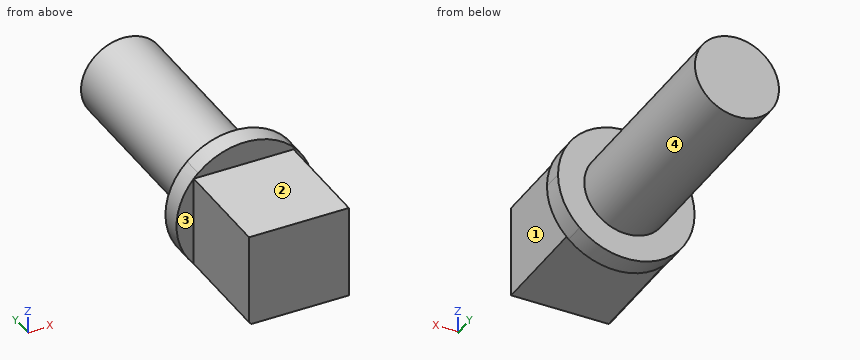
```python
from build123d import *

# Parameters (mm, degrees)
F0_R     = 4
F1_DEPTH = 22
F0_W     = 8.8741196746
F0_H     = 9.5
F2_DEPTH = 2
F3_DEPTH = 10
F5_DEPTH = 10


with BuildPart() as f1:
    # F0 (on Front) → F1 (new body)
    with BuildSketch(Plane.XZ):
        Circle(F0_R)
    extrude(amount=-F1_DEPTH)

    # F0 (on Front) → F2 (join)
    with BuildSketch(Plane.XZ):
        with BuildLine():
            ThreePointArc((4.4370598373, -4.75), (5.9620000395, -2.5893156487), (6.5, 0))
            ThreePointArc((6.5, 0), (5.9620000395, 2.5893156487), (4.4370598373, 4.75))
            Line((4.4370598373, 4.75), (4.4370598373, -4.75))
        make_face()
        with BuildLine():
            Line((-4.4370598373, 4.75), (4.4370598373, 4.75))
            ThreePointArc((4.4370598373, 4.75), (0, 6.5), (-4.4370598373, 4.75))
        make_face()
        Rectangle(F0_W, F0_H)
        Circle(F0_R, mode=Mode.SUBTRACT)
        with BuildLine():
            ThreePointArc((-4.4370598373, -4.75), (0, -6.5), (4.4370598373, -4.75))
            Line((4.4370598373, -4.75), (-4.4370598373, -4.75))
        make_face()
        with BuildLine():
            Line((-4.4370598373, -4.75), (-4.4370598373, 4.75))
            ThreePointArc((-4.4370598373, 4.75), (-6.5, 0), (-4.4370598373, -4.75))
        make_face()
    extrude(amount=-F2_DEPTH)

    # F3 (add): a face of the model
    f3_faces = [f1.faces().sort_by_distance(p)[0] for p in [
        (0, 0, 0),
    ]]
    extrude(f3_faces, amount=F3_DEPTH)

    # F4 (on face) → F5 (cut)
    with BuildSketch(Plane.XZ.offset(10)):
        with BuildLine():
            ThreePointArc((6.5, 0), (2.3093271481, 6.0759368103), (-4.8590794225, 4.3173310234))
            Line((-4.8590794225, 4.3173310234), (4.6409205775, 4.3173310234))
            Line((4.6409205775, 4.3173310234), (4.6409205775, -4.551028037))
            ThreePointArc((4.6409205775, -4.551028037), (6.0173076934, -2.4580496584), (6.5, 0))
        make_face()
        with BuildLine():
            ThreePointArc((-4.6409205775, -4.551028037), (0, -6.5), (4.6409205775, -4.551028037))
            Line((4.6409205775, -4.551028037), (-4.6409205775, -4.551028037))
        make_face()
        with BuildLine():
            Line((-4.8590794225, -4.3173310234), (-4.8590794225, 4.3173310234))
            ThreePointArc((-4.8590794225, 4.3173310234), (-6.5, 0), (-4.8590794225, -4.3173310234))
        make_face()
    extrude(amount=-F5_DEPTH, mode=Mode.SUBTRACT)


solid = f1.part
```
Source: CAD feature listing. Evaluate the final solid. Frame: model axes, mm. Face numbers are marked on the shaded views. A direction names the side the tool comes from. Coordinates: 2 decimals unless noted, no trailing zeros. Write each loop counter-clockwise with the first axis right and the second up, starting at its lowest first coordinate (ties: lowest second). Pieces come first, ordered by that corner, then holes. Notation, with made-up numbers: (28.25, 83) -> (63.25, 83) arc R28 ccw to (63.25, 101) -> close; hole circle Ø8 at (31.25, 33.5). An arc over 180 degrees is marked (long way). Return JSON: item names as keys, results as strings. Group by question number.
1) Contact query for flat-ended pins moving along their axis: P1, Ø4, axis at x = 5, z = -5, coming from the +Y side; P2, Ø4, axis at y = 11.5, z = 2.5, coming from the +X side; P3, Ø1.5, axis at y = 3, z = -2.5, coming from the +X side. Output: stop coordinate, or through.
2) Section query A-A, the plane x = 0. Return loops of the section in (y, z).
3) Section query B-B, the plane y = -6.5. Return loops of the section in (x, z).
4) Set-up query: the marked faces 1, 2, 3 and 4. Return all of +Z, -Z, +X, -X, +Y, -Y with unobstructed straight access to the full face (end or side cutting, diameter ignored); none if empty.
5) Section query C-C, the plane z = 2. Return loops of the section in (x, y).
6) Section query D-D, the plane y = 9.5. Return loops of the section in (x, z), plus the area to 3 significant figures.
7) Ray query, line 1 along Y through (x, z) = (-4.5, -4); line 2 along Z through (x, y) = (4.5, -8); line 3 along Z through (x, y) = (-0.25, 14). Return the intervals inside material, ascending.
From the geometry:
{
 "1": {"P1": "y = 2", "P2": "x = 3.97", "P3": "x = 3.6"},
 "2": {"outline": "(-10, -4.55) -> (0, -4.55) -> (0, -6.5) -> (2, -6.5) -> (2, -4) -> (22, -4) -> (22, 4) -> (2, 4) -> (2, 6.5) -> (0, 6.5) -> (0, 4.32) -> (-10, 4.32) -> close"},
 "3": {"outline": "(-4.86, -4.32) arc R6.5 ccw to (-4.64, -4.55) -> (4.64, -4.55) -> (4.64, 4.32) -> (-4.86, 4.32) -> close"},
 "4": {"face 1": "+Z, -Z, +X, -Y", "face 2": "+Z, +X, -X, -Y", "face 3": "+Z, -Z, -X, -Y", "face 4": "+Y"},
 "5": {"outline": "(-6.18, 0) -> (-4.86, 0) -> (-4.86, -10) -> (4.64, -10) -> (4.64, 0) -> (6.18, 0) -> (6.18, 2) -> (3.46, 2) -> (3.46, 22) -> (-3.46, 22) -> (-3.46, 2) -> (-6.18, 2) -> close"},
 "6": {"outline": "circle Ø8 at (0, 0)", "area": "50.3 mm²"},
 "7": {"line 1": "-10 to 2", "line 2": "-4.55 to 4.32", "line 3": "-3.99 to 3.99"}
}
